Input: part model. Units: mm. Frame: model coordinates. A direction names the side the tool comes from. Coordinates: 2 decimals unless noted, no trailing zeros. Order: outer loops, then holes, each group sorted by start corner. A loop starts at its lowest first (then second) coordinate and runs counter-clockwise, first axis right, second up.
from build123d import *

# Parameters (mm, degrees)
SKETCH1_R           = 6.35
BOSS_EXTRUDE1_DEPTH = 51
CUT_EXTRUDE1_DEPTH  = 35
SKETCH3_R           = 1.5
CUT_EXTRUDE2_DEPTH  = 15


with BuildPart() as part:
    # Sketch1 → Boss-Extrude1 (new, symmetric)
    with BuildSketch(Plane.XY):
        Circle(SKETCH1_R)
    extrude(amount=BOSS_EXTRUDE1_DEPTH, both=True)

    # Sketch2 → Cut-Extrude1 (cut)
    with BuildSketch(Plane.XY.offset(51)):
        with BuildLine():
            ThreePointArc((5.596650784, 3), (0, 6.35), (-5.596650784, 3))
            Line((-5.596650784, 3), (5.596650784, 3))
        make_face()
        with BuildLine():
            Line((5.596650784, -3), (-5.596650784, -3))
            ThreePointArc((-5.596650784, -3), (0, -6.35), (5.596650784, -3))
        make_face()
    extrude(amount=-CUT_EXTRUDE1_DEPTH, mode=Mode.SUBTRACT)

    # Sketch3 → Cut-Extrude2 (cut)
    with BuildSketch(Plane(origin=(0, 3, 0), x_dir=(1, 0, 0), z_dir=(0, 1, 0))):
        with Locations(Location((0, -21.732039108, 0), (0, 0, 90))):
            Circle(SKETCH3_R)
        with Locations(Location((0, -34.232039108, 0), (0, 0, 90))):
            Circle(SKETCH3_R)
        with Locations(Location((0, -46.732039108, 0), (0, 0, 90))):
            Circle(SKETCH3_R)
    extrude(amount=-CUT_EXTRUDE2_DEPTH, mode=Mode.SUBTRACT)


solid = part.part
Item 1: Draft query along Z for faces 1 (the face through (0, 4, 16)), 2 (the face through (6.057, 1.907, -10.619)), 3 (the face through (0.913, 0.042, 47.922)). Return one class per face: pulls with the +Z half, pulls with the -Z half, needs draft (parallel to the pull), parting line crosses it, or undercut.
Response values:
face 1: pulls with the +Z half
face 2: needs draft
face 3: undercut
Item 2: Cut plane A-A on x = 0. Return loops of the section in (y, z).
Response values:
outline: (-6.35, -51) - (6.35, -51) - (6.35, 16) - (3, 16) - (3, 20.23) - (-3, 20.23) - (-3, 16) - (-6.35, 16) - close; (-3, 23.23) - (3, 23.23) - (3, 32.73) - (-3, 32.73) - close; (-3, 35.73) - (3, 35.73) - (3, 45.23) - (-3, 45.23) - close; (-3, 48.23) - (3, 48.23) - (3, 51) - (-3, 51) - close
Item 3: Cut plane D-D on y = 5.5. Return loops of the section in (x, z), then the cut area to 3 significant figures.
Response values:
outline: (-3.17, -51) - (3.17, -51) - (3.17, 16) - (-3.17, 16) - close
area: 425 mm2
Item 4: Cut plane C-C on z = -4. Return loops of the section in (x, y), then the cut area to 3 significant figures.
Response values:
outline: circle Ø12.7 at (0, 0)
area: 127 mm2
Item 5: Pin query (flat end, axial travel): pin 1 Ø1 at (x, y) = (1.5, -5.5) entering from +Z; pin 2 Ø2 at (y, z) = (-4.5, -26) entering from -X; pin 3 Ø4 at (x, z) = (0, 46.73) entering from -Y; pin 4 Ø2.5 at (x, z) = (0, 21.73) entering from -Y. Return the tip coordinate at first contact, or that it passes through.
Response values:
pin 1: stops at z = 16
pin 2: stops at x = -5.3
pin 3: stops at y = -3
pin 4: passes through
Item 6: Ray query, probe 1 along Z at (x, y) = (0.5, -2.5); probe 2 along Y at (x, z) = (-2.25, 27); probe 3 along Y at (x, z) = (-0.5, -39). Return the intervals inside material, ascending.
Response values:
probe 1: z = -51 to 20.32, 23.15 to 32.82, 35.65 to 45.32, 48.15 to 51
probe 2: y = -3 to 3
probe 3: y = -6.33 to 6.33
Item 7: Cut plane B-B on y = 0. Return loops of the section in (x, z), then the cut area to 3 significant figures.
Response values:
outline: (-6.35, -51) - (6.35, -51) - (6.35, 51) - (-6.35, 51) - close; hole circle Ø3 at (0, 21.73); hole circle Ø3 at (0, 34.23); hole circle Ø3 at (0, 46.73)
area: 1,270 mm2
Item 8: Access query for faces 4 (the face through (-0.07, 0.04, 23.23)), 5 (the face through (2, 3, 34)), 6 (the face through (0, -4, 16)). Directions: +Z, -Z, +X, -X, +Y, -Y. A direction counts if a zero-diameter tool reaches every point of the face in a straight line with its end or side. Return the directions, or none.
Response values:
face 4: +Y, -Y
face 5: +Z, +X, -X, +Y
face 6: +Z, +X, -X, -Y
